CAD build for the part. Positions are in the model's coordinates, mm. Face numbers are marked on the shaded views. A direction names the side the tool comes from. Give positions to 0.01 mm unless a question says otherwise; leave off trailing zeros. Order: outer loops, then holes, each group sorted by start corner. A loop starts at its lowest first (then second) coordinate and runs counter-clockwise, first axis right, second up.
Item 1: Flat gauge pins, fed straight in: P1, Ø5, axis at x = 3.5, z = -4.5, coming from the -Y side; P2, Ø3, axis at x = -3.5, z = -4, coming from the -Y side; P3, Ø3, axis at x = -2.5, z = -2.5, coming from the +Y side; P4, Ø4.5, axis at x = 0, y = 0, coming from the -Z side. Where does each tip first touch, or does it go through?
Item 2: Band-saw the part on D-D on z = -4.5. Give the cut face in (x, y).
Item 3: Wall check: L1, parallel to Y at x = 0, z = -7; L2, parallel to Y at x = 0, z = -3; L3, parallel to Z at x = -4.75, y = -2.5. Give the ranges that are in metal, low to high.
Item 4: Two-plate mould, pull along X, no slides. Class the marked faces 1, 2 and 3: released by +X, released by -X, zero draft, split by the parting line, or undercut.
Item 5: Band-saw the part on A-A on x = 0. Give the cut face in (y, z), plus the area to 3 significant figures.
Item 6: Which spindle directions (+Z, -Z, +X, -X, +Y, -Y) get a long thin tool onto all of the face, cutting with end or side? Do the marked faces 4, 5 and 6. Say none if no direction does.
Autodesk Inventor part; units mm, degrees
ref_plane "YZ Plane" through (0, 0, 0) normal (1, 0, 0) x (0, 1, 0)
ref_plane "XZ Plane" through (0, 0, 0) normal (0, 1, 0) x (-1, 0, 0)
ref_plane "XY Plane" through (0, 0, 0) normal (0, 0, 1) x (1, 0, 0)
sketch "Sketch1" plane through (0, 0, 0) normal (0, 0, 1) x (1, 0, 0)
  circle A0 centre (0, 0) radius 4.8415
  dimension "d0" = 9.6831
extrude "Extrusion1" add sketch "Sketch1" along normal mid plane 7.5
sketch "Sketch2" plane through (0, 0, 3.75) normal (0, 0, 1) x (1, 0, 0)
  circle A0 centre (0, 0) radius 4.8415
  circle A1 centre (0, 4.8415) radius 0.795
  dimension "d4" = 1.59
extrude "Extrusion2" cut sketch "Sketch2" against normal through all contours A1 A0 | A0 A1 picked at (0, 4.5717) picked at (0.0219, 5.1007)
pattern_circular "Circular Pattern1" count 16 over 360 about axis through (0, 0, 0) along (0, 0, 1) of "Extrusion2"
sketch "Sketch3" plane through (0, 0, 3.75) normal (0, 0, 1) x (1, 0, 0)
  arc A0 (2.8171, 3.9376) -> (2.5598, 4.1095) centre (0, 0) ccw
  circle A1 centre (0, 0) radius 6.5
  dimension "d11" = 13
extrude "Extrusion3" add sketch "Sketch3" along normal blind 1
sketch "Sketch4" plane through (0, 0, -3.75) normal (0, 0, -1) x (-1, 0, 0)
  circle A0 centre (0, 0) radius 6.5
extrude "Extrusion4" add sketch "Sketch4" along normal blind 7
sketch "Sketch5" plane through (0, 0, -10.75) normal (0, 0, -1) x (-1, 0, 0)
  circle A0 centre (0, 0) radius 6.5
  circle A1 centre (0, 0) radius 2.5
  dimension "d17" = 5
extrude "Extrusion5" cut sketch "Sketch5" against normal through all contours A1
chamfer "Chamfer1" distance 0.25 angle 45 4 edges at (6.5, 0, -10.75) (6.5, 0, -3.75) (-6.5, 0, 3.75) (-6.5, 0, 4.75)
properties part number "drive pulley"
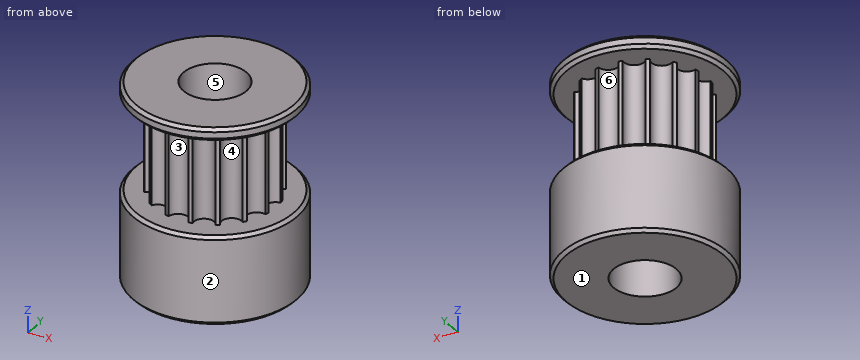
The answers:
1. P1: stops at y = -6.42
1. P2: stops at y = -6.18
1. P3: stops at y = 6.1
1. P4: passes through
2. outline: circle Ø13 at (0, 0); hole circle Ø5 at (0, 0)
3. L1: y = -6.5 to -2.5, 2.5 to 6.5
3. L2: y = -4.05 to -2.5, 2.5 to 4.05
3. L3: z = -10.75 to -3.75, 3.75 to 4.75
4. face 1: zero draft
4. face 2: split by the parting line
4. face 3: undercut
5. outline: (-6.5, -10.5) - (-6.25, -10.75) - (-2.5, -10.75) - (-2.5, 4.75) - (-6.25, 4.75) - (-6.5, 4.5) - (-6.5, 4) - (-6.25, 3.75) - (-4.05, 3.75) - (-4.05, -3.75) - (-6.25, -3.75) - (-6.5, -4) - close; (2.5, -10.75) - (6.25, -10.75) - (6.5, -10.5) - (6.5, -4) - (6.25, -3.75) - (4.05, -3.75) - (4.05, 3.75) - (6.25, 3.75) - (6.5, 4) - (6.5, 4.5) - (6.25, 4.75) - (2.5, 4.75) - close
5. area: 86.9 mm2
6. face 4: none
6. face 5: +Z, -Z
6. face 6: +Y
